from build123d import *

# Parameters (mm, degrees)
F1_DEPTH       = 5
F2_D           = 6.4
F2_CBORE_D     = 11.25
F2_CBORE_DEPTH = 2
F3_W           = 5
F3_H           = 43
F4_DEPTH       = 43
F6_D           = 3.4
F5_R           = 12.5
F7_DEPTH       = 23.001
F10_DEPTH      = 12
F11_SIZE       = 4.99999


# Not quite as in the source:
# - a fillet or chamfer is up to 0.001 mm smaller than in the source, because OpenCascade refuses the exact size
# - a feature names something its author has since deleted; it is built from what else it names


with BuildPart() as f1:
    # F0 (on Front) → F1 (new body)
    with BuildSketch(Plane.XZ):
        Polygon((0, 29), (0, 0), (80, 0), (80, 30), (75, 30), (59, 63), (59, 83), (30, 83), (30, 43), (18, 43), (18, 29), align=None)
    extrude(amount=-F1_DEPTH)

    # F2 (through all)
    with Locations(Plane.XZ):
        with Locations((10, 14.5), (44.5, 53), (44.5, 73), (70, 15)):
            CounterBoreHole(F2_D / 2, F2_CBORE_D / 2, F2_CBORE_DEPTH)

    # F3 (on face) → F4 (join)
    with BuildSketch(Plane.XZ):
        with Locations((20.5, 21.5)):
            Rectangle(F3_W, F3_H)
    extrude(amount=F4_DEPTH)

    # F6 (through all)
    with Locations(Plane.YZ.offset(23)):
        with Locations((-37, 37), (-6, 6), (-37, 6)):
            Hole(F6_D / 2)

    # F5 (on face) → F7 (cut, through all)
    with BuildSketch(Plane.YZ.offset(23)):
        with Locations((-21.5, 21.5)):
            Circle(F5_R)
    extrude(amount=-F7_DEPTH, mode=Mode.SUBTRACT)

    # F9 (on face) → F10 (cut, through all)
    with BuildSketch(Plane(origin=(18, 0, 0), x_dir=(0, -1, 0), z_dir=(-1, 0, 0))):
        Polygon((14, 43), (-5, 43), (-5, 29), (0, 29), align=None)
    extrude(amount=-F10_DEPTH, mode=Mode.SUBTRACT)

    # F11 (size 5 in the source; OpenCascade refuses exactly that, so slightly less here)
    f11_edges = [f1.edges().sort_by_distance(p)[0] for p in [
        (30, 2.5, 83),
        (59, 2.5, 83),
        (80, 2.5, 30),
        (80, 2.5, 0),
        (20.5, -43, 0),
        (0, 2.5, 0),
        (0, 2.5, 29),
        (20.5, -43, 43),
    ]]
    chamfer(f11_edges, length=F11_SIZE)


solid = f1.part
Source: CAD feature listing. Evaluate the final solid. Frame: model axes, mm. A direction names the side the tool comes from. Round coordinates to 2 decimals unless told otherwise and drop trailing zeros. Order: outer loops, then holes, each group sorted by start corner. A loop starts at its lowest first (then second) coordinate and runs counter-clockwise, first axis right, second up. Notation, with made-up numbers: (77.25, -35) -> (99.25, -35) arc R22 cw to (99.25, -18) -> close; hole circle Ø1 at (-34, -38). An arc over 180 degrees is marked (long way). Answer as CSV lines item,"result".
Item 1: Reachability of faces 4 (the face through (47.524, 0.986, 77.743)), 5 (the face through (20, -26, 43)), 6 (the face through (18, -31, 12)) from +Z, -Z, +X, -X, +Y, -Y: full face, straight path, thin tool, end or side. Return the list, or none.
A:
face 4,"-Y"
face 5,"+Z, +X, -X, +Y, -Y"
face 6,"+Z, -Z, -X, -Y"
Item 2: Section A-A, the plane y = -21.5. Return loops of the section in (x, z).
A:
outline,"(18, 0) -> (23, 0) -> (23, 9) -> (18, 9) -> close; (18, 34) -> (23, 34) -> (23, 43) -> (18, 43) -> close"
Item 3: Section C-C, the plane z = 6. Return loops of the section in (x, y), plus the area to 3 significant figures.
A:
outline,"(0, 0) -> (18, 0) -> (18, -4.3) -> (23, -4.3) -> (23, 0) -> (80, 0) -> (80, 5) -> (0, 5) -> close; (18, -43) -> (23, -43) -> (23, -38.7) -> (18, -38.7) -> close; (18, -35.3) -> (23, -35.3) -> (23, -7.7) -> (18, -7.7) -> close"
area,"581 mm²"
Item 4: Pin query (flat end, axial travel): pin 1 Ø1.5 at (y, z) = (3.5, 73.5) entering from +X; pin 2 Ø2.5 at (x, y) = (15.5, 2) entering from +Z; pin 3 Ø2.5 at (y, z) = (1.5, 53) entering from -X. Return the tip coordinate at first contact, or that it passes through.
A:
pin 1,"x = 59"
pin 2,"z = 29"
pin 3,"x = 30"
Item 5: Line query: L1, parallel to Z at x = 10, y = 1.2 (3 decimals); L2, parallel to X at y = -24.5, z = 7.5; L3, parallel to Y at x = 60, z = 46.5. Output: solid intervals per line, ascending.
A:
L1,"0 to 8.875, 20.125 to 29"
L2,"18 to 23"
L3,"0 to 5"
Item 6: Section B-B, the plane y = -37. Return loops of the section in (x, z), plus the area to 3 significant figures.
A:
outline,"(18, 0) -> (23, 0) -> (23, 4.3) -> (18, 4.3) -> close; (18, 7.7) -> (23, 7.7) -> (23, 35.3) -> (18, 35.3) -> close; (18, 38.7) -> (23, 38.7) -> (23, 43) -> (18, 43) -> close"
area,"181 mm²"
Item 7: Section D-D, the plane z = 53. Return loops of the section in (x, y) (3 decimals).
A:
outline,"(30, 0) -> (38.875, 0) -> (38.875, 2) -> (41.3, 2) -> (41.3, 5) -> (30, 5) -> close; (47.7, 2) -> (50.125, 2) -> (50.125, 0) -> (63.848, 0) -> (63.848, 5) -> (47.7, 5) -> close"
Item 8: Pull-direction query (Z, two-part tool) for faces 1 (the face through (3, 2, 27)), 2 (the face through (0, 2, 15)), 3 (the face through (10.694, 3.521, 11.376)); classes: pulls with the +Z half, pulls with the -Z half, needs draft (parallel to the pull), parting line crosses it, or undercut.
A:
face 1,"pulls with the +Z half"
face 2,"needs draft"
face 3,"undercut"
